Model file for the job. Use its own axes, mm. Give positions to 0.01 mm unless a question says otherwise; leave off trailing zeros. Order: outer loops, then holes, each group sorted by start corner. A loop starts at its lowest first (then second) coordinate and runs counter-clockwise, first axis right, second up. Notation, with made-up numbers: (69.25, 88.25) - (113.25, 88.25) arc R24 cw to (113.25, 107.25) - close; hole circle Ø4 at (14, 33.5). An arc over 180 degrees is marked (long way). Use CSV: the item, a comma, the result in double quotes. Start each with the question number.
(1) Probe L1, parallel to Y at x = 2.25, z = 37; L2, parallel to Z at x = 3.25, y = 240; L3, parallel to Z at x = 0.5, y = 143.5. List the from-to ranges inside material, lowest first.
(2) Band-saw the part on D-D, the plane y = 69.5. Give the cut face in (x, z).
(3) Band-saw the part on C-C, the plane z = 680. Give the cut face in (x, y).
(4) Band-saw the part on B-B, the plane x = 2. Count the separate pieces of the cut face and the enclosed holes in it, then the cut area to 3 significant figures.
(5) Drop flat-ended pins along their axis: pin 1 Ø3 at (x, z) = (3, 28.5) entering from +Y; pin 2 Ø3 at (x, y) = (3, 464.5) entering from +Z; pin 3 Ø12 at (y, z) = (315, 533) entering from +X; pin 4 Ø5 at (x, y) = (4.5, 382) entering from -Z. Give the stop position or say it passes through.
(6) Band-saw the part on A-A, the plane z = 172.5. Give the cut face in (x, y).
from build123d import *

# Parameters (mm, degrees)
PAD_DEPTH       = 10
SKETCH001_W     = 10
SKETCH001_H     = 50
SKETCH001_W_2   = 50
SKETCH001_H_2   = 10
POCKET_DEPTH    = 10.001
POCKET001_DEPTH = 10.001


with BuildPart() as part:
    # Sketch → Pad (new body)
    with BuildSketch(Plane.YZ):
        with BuildLine():
            Line((0, 0), (458.57, 0))
            Line((458.57, 50), (458.57, 0))
            Line((468.57, 50), (458.57, 50))
            Line((468.57, 323.200359), (468.57, 50))
            Line((458.57, 323.200359), (468.57, 323.200359))
            Line((458.57, 373.200359), (458.57, 323.200359))
            Line((468.57, 373.200359), (458.57, 373.200359))
            Line((468.57, 646.400718), (468.57, 373.200359))
            Line((458.57, 646.400718), (468.57, 646.400718))
            Line((458.57, 696.400718), (458.57, 646.400718))
            Line((468.57, 696.400718), (458.57, 696.400718))
            ThreePointArc((468.57, 696.400718), (465.136205, 705.951787), (456.406946, 711.13))
            Line((456.406946, 711.13), (354.229363, 730.81))
            ThreePointArc((354.229363, 730.81), (342.983266, 728.501917), (336.663136, 718.917664))
            Line((336.663136, 718.917664), (315.777541, 610.480692))
            ThreePointArc((-15, 86.92), (258.192075, 280.591887), (315.777541, 610.480692))
            Line((-15, 15), (-15, 86.92))
            ThreePointArc((-15, 15), (-10.606602, 4.393398), (0, 0))
        make_face()
    extrude(amount=PAD_DEPTH)

    # Sketch001 → Pocket (cut, through all)
    with BuildSketch(Plane.YZ.offset(10)):
        Polygon((276.869428, 134.731244), (285.551837, 183.971631), (295.399915, 182.235149), (286.717506, 132.994762), align=None)
        Polygon((313.682842, 343.510487), (322.365251, 392.750875), (332.213328, 391.014393), (323.530919, 341.774005), align=None)
        Polygon((359.178664, 601.530119), (350.496255, 552.289731), (360.344333, 550.553249), (369.026742, 599.793637), align=None)
        Polygon((101.965072, 100.867809), (151.379199, 108.499589), (152.905555, 98.616763), (103.491428, 90.984984), align=None)
        Polygon((235.976184, 121.565195), (285.390311, 129.196975), (286.916667, 119.31415), (237.50254, 111.68237), align=None)
        with Locations((118.247, 45.35)):
            Rectangle(SKETCH001_W, SKETCH001_H)
        with Locations((238.247, 5)):
            Rectangle(SKETCH001_W_2, SKETCH001_H_2)
        with Locations((388.247, 5)):
            Rectangle(SKETCH001_W_2, SKETCH001_H_2)
    extrude(amount=-POCKET_DEPTH, mode=Mode.SUBTRACT)

    # Sketch002 → Pocket001 (cut, through all)
    with BuildSketch(Plane.YZ.offset(10)):
        Polygon((422.310473, 703.463594), (373.212868, 712.92008), (371.321571, 703.100559), (420.419176, 693.644073), align=None)
        Polygon((315.96561, 609.813), (325.785131, 607.921703), (323.893833, 598.102182), (314.074312, 599.993479), align=None)
    extrude(amount=-POCKET001_DEPTH, mode=Mode.SUBTRACT)


solid = part.part
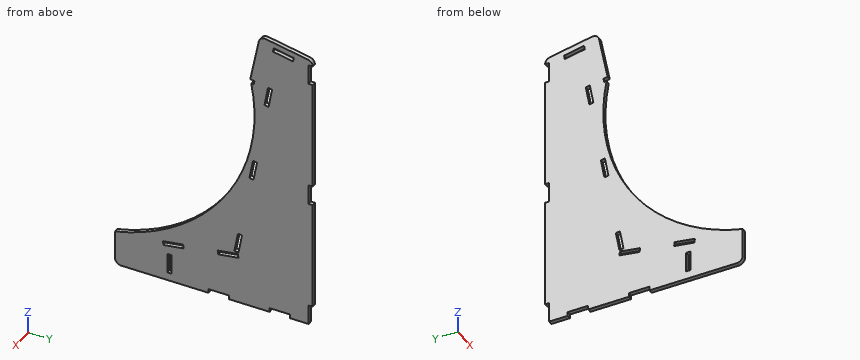
Answer block:
1,L1,"y = -15 to 113.25, 123.25 to 458.57"
1,L2,"z = 10 to 112.07, 122.19 to 254.01"
1,L3,"z = 0 to 97.16, 107.28 to 158.69"
2,outline,"(0, 0) - (10, 0) - (10, 115.65) - (0, 115.65) - close"
3,outline,"(0, 329.17) - (10, 329.17) - (10, 458.57) - (0, 458.57) - close"
4,separate pieces,"1"
4,enclosed holes,"7"
4,area,"164,000 mm2"
5,pin 1,"stops at y = 458.57"
5,pin 2,"stops at z = 708.07"
5,pin 3,"passes through"
5,pin 4,"stops at z = 10"
6,outline,"(0, 161.65) - (10, 161.65) - (10, 283.53) - (0, 283.53) - close; (0, 293.68) - (10, 293.68) - (10, 468.57) - (0, 468.57) - close"
